Autodesk Inventor part; units mm, degrees
ref_plane "Work Plane1" through (0, 0, 4.318) normal (0, 0, -1) x (-1, 0, 0)
ref_plane "YZ Plane" through (0, 0, 0) normal (1, 0, 0) x (0, 1, 0)
ref_plane "XZ Plane" through (0, 0, 0) normal (0, 1, 0) x (-1, 0, 0)
sketch "Sketch1" plane through (0, 0, 0) normal (0, 0, 1) x (1, 0, 0)
  line L0 (0, 11.43) -> (0, -11.43)
  line L1 (0, 13.081) -> (-66.04, 13.081)
  line L2 (-66.04, 13.081) -> (-66.04, -13.081)
  line L3 (-66.04, -13.081) -> (0, -13.081)
  line L4 (0, -13.081) -> (0, 13.081)
  point P0 (0, 0)
  point P1 (0, 0)
  dimension "d1" = 26.162
  dimension "d3" = 66.04
extrude "Extrusion1" add sketch "Sketch1" along normal blind 160.02
ref_plane "Work Plane1" through (0, 0, 4.318) normal (0, 0, -1) x (-1, 0, 0)
sketch "Sketch3" plane through (0, 0, 4.318) normal (0, 0, -1) x (-1, 0, 0)
  line L0 (0, 13.081) -> (-68.58, 13.081)
  line L1 (-68.58, 13.081) -> (-68.58, -9.779)
  line L2 (-68.58, -9.779) -> (0, -9.779)
  line L3 (0, -9.779) -> (0, 13.081)
  line L4 (0, -13.081) -> (0, 13.081)
  line L5 (66.04, 13.081) -> (66.04, -13.081)
  line L6 (0, 13.081) -> (66.04, 13.081)
  point P0 (0, 0)
  point P1 (0, 0)
  dimension "d13" = 22.86
  dimension "d14" = 134.62
extrude "Extrusion3" add sketch "Sketch3" against normal blind 151.384
fillet "Fillet1" radius 1.27 6 edges at (34.29, -9.779, 4.318) (68.58, -9.779, 80.01) (34.29, -9.779, 155.702) (0, -9.779, 80.01) (0, 1.651, 155.702) (0, 1.651, 4.318)
properties part number "BatteryInBag"
Input: part model. Units: mm. Frame: model coordinates. A direction names the side the tool comes from. Coordinates: 2 decimals unless noted, no trailing zeros. Write each loop counter-clockwise with the first axis right and the second up, starting at its lowest first coordinate (ties: lowest second). Pieces come first, ordered by that corner, then holes. Notation, with made-up numbers: M 40.5,-7.75 L 77.5,-7.75 A11 ccw 77.5,12.25 Z; hole C 78.25,-18.75 d2. An arc over 180 degrees is marked long. Use one line per item in the form item = value.
Q1. Set-up query: faces 1 (the face through (-33, -13.081, 79)), 2 (the face through (35, -9.779, 79)), 3 (the face through (35, 2, 4.318)), 4 (the face through (-33, 0, 0)), 5 (the face through (35, 2, 155.702)). Return all of +Z, -Z, +X, -X, +Y, -Y with unobstructed straight access to the full face (end or side cutting, diameter ignored); none if empty.
Answer below:
face_1 = +Z, -Z, +X, -X, -Y
face_2 = +Z, -Z, +X, -Y
face_3 = -Z, +X, +Y, -Y
face_4 = -Z, +X, -X, +Y, -Y
face_5 = +Z, +X, +Y, -Y
Q2. Material intervals for probe 1 along Y at (x, z) = (29.5, 63); probe 2 along Z at (x, y) = (37, -8.5); probe 3 along X at (y, z) = (-12, 27.5), sorted ascending. Write a range as from..to.
Answer below:
probe_1 = -9.78..13.08
probe_2 = 4.32..155.7
probe_3 = -66.04..0
Q3. Section A-A (x = 43). Return loops of the section in (y, z).
Answer below:
outline = M -9.78,5.59 A1.27 ccw -8.51,4.32 L 13.08,4.32 L 13.08,155.7 L -8.51,155.7 A1.27 ccw -9.78,154.43 Z
Q4. Section C-C (z = 62). Return loops of the section in (x, y), plus the area to 3 significant figures.
Answer below:
outline = M -66.04,-13.08 L 0,-13.08 L 0,-11.05 A1.27 cw 1.27,-9.78 L 67.31,-9.78 A1.27 ccw 68.58,-8.51 L 68.58,13.08 L -66.04,13.08 Z
area = 3,300 mm²
Q5. Section B-B (y = 5.5). Return loops of the section in (x, z).
Answer below:
outline = M -66.04,0 L 0,0 L 0,3.05 A1.27 cw 1.27,4.32 L 68.58,4.32 L 68.58,155.7 L 1.27,155.7 A1.27 cw 0,156.97 L 0,160.02 L -66.04,160.02 Z
Q6. First-contact query: pin 1 (1.5 mm diameter, centred on x = 31, y = 9, fed in from -Z); pin 2 (20 mm diameter, centred on x = 27.5, z = 85, fed in from -Y); pin 3 (8 mm diameter, centred on x = 25, y = 3, fed in from +Z). Flat tips, straight axial feed; report the tip coordinate or a pass-through.
Answer below:
pin_1 = 4.32
pin_2 = -9.78
pin_3 = 155.7
